Part print with two shaded views. Sizes in mm from the minimum x, y, z corner. Coordinates: 2 decimals unless noted, no trailing zeros. Loops run counter-clockwise (first coordinate to the right, second up) from the corner with the lowest first, then second, coordinate; pieces in that order, holes last.
Item 1: Cut at A-A (x = 10). List the corners of the cut face in (y, z).
Item 2: Drill centre lines: line 1 along Y through (x, z) = (10, 1.7); line 2 along X through (y, z) = (43.5, 2.7); line 3 along Y through (x, z) = (23, 0.3). Where is each one in solid material? Low to high.
Item 3: Cut at B-B (y = 84.75). List the corners of the cut face in (x, z).
Item 4: Cut at D-D (x = 25). List the corners of the cut face in (y, z).
Item 5: Cut at C-C (z = 2.2). List the corners of the cut face in (x, y), and give its area (3 significant figures).
Item 6: Flat gauge pins, fed straight in: pin 1 (3 mm diameter, centred on x = 70, y = 11.25, fed in from -Z); pin 2 (0.9 mm diameter, centred on y = 94, z = 2, fed in from -X); pin 3 (0.9 mm diameter, centred on y = 48.5, z = 2, fed in from +X); pin 4 (0.9 mm diameter, centred on x = 55, z = 1, fed in from +Y). Where does each tip first touch, or does it go through?
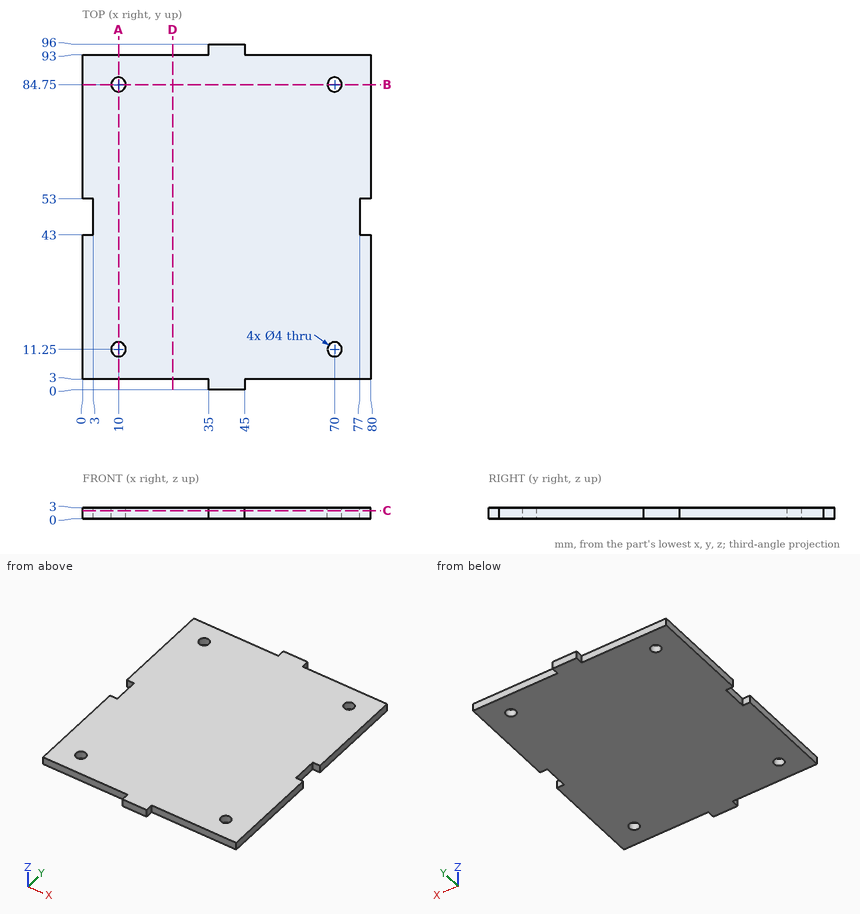
Filled sheet:
1. outline: (3, 0) - (9.25, 0) - (9.25, 3) - (3, 3) - close; (13.25, 0) - (82.75, 0) - (82.75, 3) - (13.25, 3) - close; (86.75, 0) - (93, 0) - (93, 3) - (86.75, 3) - close
2. line 1: y = 3 to 9.25, 13.25 to 82.75, 86.75 to 93
2. line 2: x = 3 to 77
2. line 3: y = 3 to 93
3. outline: (0, 0) - (8, 0) - (8, 3) - (0, 3) - close; (12, 0) - (68, 0) - (68, 3) - (12, 3) - close; (72, 0) - (80, 0) - (80, 3) - (72, 3) - close
4. outline: (3, 0) - (93, 0) - (93, 3) - (3, 3) - close
5. outline: (0, 3) - (35, 3) - (35, 0) - (45, 0) - (45, 3) - (80, 3) - (80, 43) - (77, 43) - (77, 53) - (80, 53) - (80, 93) - (45, 93) - (45, 96) - (35, 96) - (35, 93) - (0, 93) - (0, 53) - (3, 53) - (3, 43) - (0, 43) - close; hole circle Ø4 at (10, 11.25); hole circle Ø4 at (10, 84.75); hole circle Ø4 at (70, 11.25); hole circle Ø4 at (70, 84.75)
5. area: 7,150 mm2
6. pin 1: passes through
6. pin 2: stops at x = 35
6. pin 3: stops at x = 77
6. pin 4: stops at y = 93
